from build123d import *

# Parameters (mm, degrees)
BOSS_EXTRUDE1_DEPTH = 44
SKETCH2_W           = 40
SKETCH2_H           = 36
CUT_EXTRUDE1_DEPTH  = 87.219887541
SKETCH3_R           = 0.75
CUT_EXTRUDE2_DEPTH  = 99.468948566


with BuildPart() as part:
    # Sketch1 → Boss-Extrude1 (new body)
    with BuildSketch(Plane.XY):
        with BuildLine():
            Line((25.485483108, -5.097096622), (25.093250837, -7.058257973))
            Line((25.093250837, -7.058257973), (28.996154216, -7.838838649))
            Line((28.996154216, -7.838838649), (28.996154216, -22.083484054))
            ThreePointArc((28.996154216, -22.083484054), (19.496154216, -31.583484054), (28.996154216, -41.083484054))
            Line((28.996154216, -41.083484054), (28.996154216, -52.083484054))
            Line((28.996154216, -52.083484054), (24.996154216, -52.083484054))
            Line((24.996154216, -52.083484054), (24.996154216, -54.083484054))
            Line((24.996154216, -54.083484054), (74.219381244, -54.083484054))
            Line((74.219381244, -54.083484054), (74.219381244, -52.083484054))
            Line((74.219381244, -52.083484054), (70.219381244, -52.083484054))
            Line((70.219381244, -52.083484054), (70.219381244, -39.083484054))
            Line((70.219381244, -39.083484054), (68.219381244, -39.083484054))
            ThreePointArc((68.219381244, -39.083484054), (60.719381244, -31.583484054), (68.219381244, -24.083484054))
            Line((68.219381244, -24.083484054), (70.219381244, -24.083484054))
            Line((70.219381244, -24.083484054), (70.219381244, -20.083484054))
            Line((70.219381244, -20.083484054), (70.219381244, -16.083484054))
            Line((70.219381244, -16.083484054), (74.122284622, -16.86406473))
            Line((74.122284622, -16.86406473), (74.514516892, -14.902903378))
            Line((74.514516892, -14.902903378), (64.708710135, -12.941742027))
            Line((64.708710135, -12.941742027), (64.316477865, -14.902903378))
            Line((64.316477865, -14.902903378), (68.219381244, -15.683484054))
            Line((68.219381244, -15.683484054), (68.219381244, -22.083484054))
            ThreePointArc((68.219381244, -22.083484054), (58.719381244, -31.583484054), (68.219381244, -41.083484054))
            Line((68.219381244, -41.083484054), (68.219381244, -52.083484054))
            Line((68.219381244, -52.083484054), (30.996154216, -52.083484054))
            Line((30.996154216, -52.083484054), (30.996154216, -39.083484054))
            Line((30.996154216, -39.083484054), (28.996154216, -39.083484054))
            ThreePointArc((28.996154216, -39.083484054), (21.496154216, -31.583484054), (28.996154216, -24.083484054))
            Line((28.996154216, -24.083484054), (30.996154216, -24.083484054))
            Line((30.996154216, -24.083484054), (30.996154216, -8.238838649))
            Line((30.996154216, -8.238838649), (34.899057594, -9.019419324))
            Line((34.899057594, -9.019419324), (35.291289865, -7.058257973))
            Line((35.291289865, -7.058257973), (25.485483108, -5.097096622))
        make_face()
    extrude(amount=-BOSS_EXTRUDE1_DEPTH)

    # Sketch2 → Cut-Extrude1 (cut, through all)
    with BuildSketch(Plane(origin=(70.219381244, 0, 0), x_dir=(0, 0, -1), z_dir=(1, 0, 0))):
        with Locations((22, -34.083484054)):
            Rectangle(SKETCH2_W, SKETCH2_H)
    extrude(amount=-CUT_EXTRUDE1_DEPTH, mode=Mode.SUBTRACT)

    # Sketch3 → Cut-Extrude2 (cut, through all)
    with BuildSketch(Plane(origin=(0, -52.083484054, 0), x_dir=(1, 0, 0), z_dir=(0, 1, 0))):
        with Locations(Location((49.60776773, 39, 0), (0, 0, 180))):
            Circle(SKETCH3_R)
        with Locations(Location((49.60776773, 5, 0), (0, 0, 180))):
            Circle(SKETCH3_R)
    extrude(amount=-CUT_EXTRUDE2_DEPTH, mode=Mode.SUBTRACT)


solid = part.part
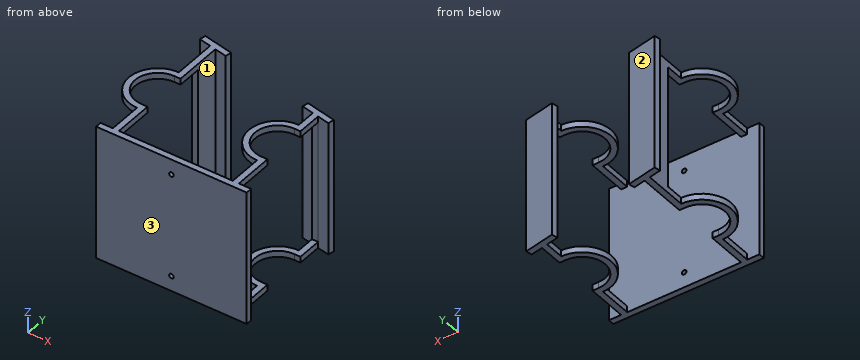
Source: CAD feature listing. Evaluate the final solid. Frame: model axes, mm. Face numbers are marked on the shaded views. Round coordinates to 2 decimals unless told otherwise and drop trailing zeros. Loops run counter-clockwise (first coordinate to the right, second up) from the corner with the lowest first, then second, coordinate; pieces in that order, holes last. Notation, with made-up numbers: M 23.5,-10.75 L 37.5,-10.75 A17 cw 37.5,-2.75 Z; hole C 65,68 d9. An arc over 180 degrees is marked long. Return JSON: item names as keys, results as strings. Group by question number.
1. Mould query, pull axis Y, two halves, no side actions, for the marked faces 1, 2 and 3. Classes: released by +Y, released by -Y, zero draft, split by the parting line, or undercut.
2. Section query A-A on y = -20. Output: boundary loops of the cut face in (x, z), and give its area (3 significant figures).
3. Section query D-D on z = -39. Output: boundary loops of the cut face in (x, y), and give its area (3 significant figures).
4. Pin query (flat end, axial travel): pin 1 (0.6 mm diameter, centred on y = -53.5, z = -33, fed in from +X); pin 2 (1.6 mm diameter, centred on y = -47, z = -1, fed in from +X); pin 3 (1 mm diameter, centred on y = -49, z = -43, fed in from -X); pin 4 (12 mm diameter, centred on x = 27, y = -36.5, fed in from +Z). Return the tip coordinate at first contact, or that it passes through.
5. Material intervals for line 1 along X through (y, z) = (-53.55, -39); line 2 along Y through (x, z) = (50.5, -9.5); line 3 along Y through (x, z) = (72, -34.5), sorted ascending. Write a range as from..to.
6. Section query B-B on z = -33. Output: boundary loops of the cut face in (x, y).
7. Section query C-C on x = 30. Output: boundary loops of the cut face in (y, z).
Checks:
{
 "1": {"face 1": "undercut", "face 2": "released by +Y", "face 3": "released by -Y"},
 "2": {"outline": "M 29,-44 L 31,-44 L 31,-42 L 29,-42 Z; M 29,-2 L 31,-2 L 31,0 L 29,0 Z; M 68.22,-44 L 70.22,-44 L 70.22,-42 L 68.22,-42 Z; M 68.22,-2 L 70.22,-2 L 70.22,0 L 68.22,0 Z", "area": "16.0 mm²"},
 "3": {"outline": "M 25,-54.08 L 48.86,-54.08 L 48.86,-52.08 L 25,-52.08 Z; M 25.09,-7.06 L 29,-7.84 L 29,-16.08 L 31,-16.08 L 31,-8.24 L 34.9,-9.02 L 35.29,-7.06 L 25.49,-5.1 Z; M 50.36,-54.08 L 74.22,-54.08 L 74.22,-52.08 L 50.36,-52.08 Z; M 64.32,-14.9 L 68.22,-15.68 L 68.22,-16.08 L 70.22,-16.08 L 74.12,-16.86 L 74.51,-14.9 L 64.71,-12.94 Z", "area": "152 mm²"},
 "4": {"pin 1": "stops at x = 74.22", "pin 2": "stops at x = 70.22", "pin 3": "stops at x = 29", "pin 4": "stops at z = 0"},
 "5": {"line 1": "x = 25..48.86, 50.36..74.22", "line 2": "y = -54.08..-52.08", "line 3": "y = -54.08..-52.08, -16.44..-14.4"},
 "6": {"outline": "M 25,-54.08 L 74.22,-54.08 L 74.22,-52.08 L 25,-52.08 Z; M 25.09,-7.06 L 29,-7.84 L 29,-16.08 L 31,-16.08 L 31,-8.24 L 34.9,-9.02 L 35.29,-7.06 L 25.49,-5.1 Z; M 64.32,-14.9 L 68.22,-15.68 L 68.22,-16.08 L 70.22,-16.08 L 74.12,-16.86 L 74.51,-14.9 L 64.71,-12.94 Z"},
 "7": {"outline": "M -54.08,-44 L -39.08,-44 L -39.08,-42 L -52.08,-42 L -52.08,-2 L -39.08,-2 L -39.08,0 L -54.08,0 Z; M -24.08,-44 L -6,-44 L -6,0 L -24.08,0 L -24.08,-2 L -16.08,-2 L -16.08,-42 L -24.08,-42 Z"}
}
